from build123d import *

# Parameters (mm, degrees)
CUT_EXTRUDE1_DEPTH           = 10
CUT_REVOLVE1_ANGLE           = 157.5
CUT_REVOLVE1_OTHER_WAY_ANGLE = 157.5


with BuildPart() as part:
    # Sketch3 → Revolve1 (revolve)
    with BuildSketch(Plane.XY, mode=Mode.PRIVATE) as revolve1_sk:
        with BuildLine():
            Line((1.25, 0), (1.25, 9))
            ThreePointArc((1.25, 9), (0, 9.690197618), (-1.25, 9))
            Line((-1.25, 9), (-1.25, 0))
            Line((-1.25, 0), (1.25, 0))
        make_face()
    revolve(revolve1_sk.sketch.rotate(Axis((-1.25, 0, 0), (1, 0, 0)), 180), axis=Axis((-1.25, 0, 0), (1, 0, 0)))

    # Sketch4 → Cut-Extrude1 (cut)
    # profile 1 of 2: a face of its own
    with BuildSketch(Plane(origin=(1.25, 0, 0), x_dir=(0, 0, -1), z_dir=(1, 0, 0))):
        with BuildLine():
            Line((1.322875656, 1.5), (-1.322875656, 1.5))
            ThreePointArc((-1.322875656, 1.5), (0, -2), (1.322875656, 1.5))
        make_face()
        with BuildLine():
            ThreePointArc((-1.118033989, 1), (0, -1.5), (1.118033989, 1))
            Line((1.118033989, 1), (-1.118033989, 1))
        make_face(mode=Mode.SUBTRACT)
    # profile 2 of 2: a face of its own
    with BuildSketch(Plane(origin=(1.25, 0, 0), x_dir=(0, 0, -1), z_dir=(1, 0, 0))):
        with BuildLine():
            Line((1.118033989, 1), (-1.118033989, 1))
            ThreePointArc((-1.118033989, 1), (0, -1.5), (1.118033989, 1))
        make_face()
    extrude(amount=-CUT_EXTRUDE1_DEPTH, mode=Mode.SUBTRACT)

    # Sketch7 → Cut-Revolve1 (revolve, cut)
    with BuildSketch(Plane.XY):
        with BuildLine():
            ThreePointArc((-1.25, 9), (0, 9.690197618), (1.25, 9))
            Line((1.25, 9), (1.25, 3))
            Line((1.25, 3), (-1.25, 3))
            Line((-1.25, 3), (-1.25, 9))
        make_face()
    revolve(axis=Axis((-1.25, 0, 0), (1, 0, 0)), revolution_arc=CUT_REVOLVE1_ANGLE, mode=Mode.SUBTRACT)

    # Sketch7 → Cut-Revolve1 other way (revolve, cut)
    with BuildSketch(Plane.XY):
        with BuildLine():
            ThreePointArc((-1.25, 9), (0, 9.690197618), (1.25, 9))
            Line((1.25, 9), (1.25, 3))
            Line((1.25, 3), (-1.25, 3))
            Line((-1.25, 3), (-1.25, 9))
        make_face()
    revolve(axis=Axis((-1.25, 0, 0), (-1, 0, 0)), revolution_arc=CUT_REVOLVE1_OTHER_WAY_ANGLE, mode=Mode.SUBTRACT)


solid = part.part
Read the model definition and answer for the solid it produces. Units are mm, in the model's axes. A direction names the side the tool comes from. Coordinates: 2 decimals unless noted, no trailing zeros. Write each loop counter-clockwise with the first axis right and the second up, starting at its lowest first coordinate (ties: lowest second). Pieces come first, ordered by that corner, then holes. Notation, with made-up numbers: (-12.75, 42) - (44.25, 42) arc R15 cw to (44.25, 70) - close; hole circle Ø7 at (47.5, 40). An arc over 180 degrees is marked (long way). One line per question, with ' | ' between items.
Q1. Find section B-B, the plane y = 0. Write down the section's boundary in (x, z), plus the area to 3 significant figures.
Result set:
outline: (-1.25, -3) - (1.25, -3) - (1.25, -2) - (-1.25, -2) - close; (-1.25, 2) - (1.25, 2) - (1.25, 3) - (-1.25, 3) - close | area: 5.00 mm^2
Q2. Find section C-C, the plane x = 0.45. Write down the section's boundary in (y, z), plus the area to 3 significant figures.
Result set:
outline: (-8.89, -3.68) - (-2.77, -1.15) arc R3 ccw (long way) to (-2.77, 1.15) - (-8.89, 3.68) arc R9.62 ccw to start; hole (1.5, -1.32) - (1.5, 1.32) arc R2 ccw (long way) to start | area: 49.4 mm^2
Q3. For faces 1 (the flat face through (0, 1.5, 0)), 2 (the flat face through (0.02, -5.91, -2.45)), 3 (the flat face through (0.02, -5.91, 2.45)), determine the directions among +Z, -Z, +X, -X, +Y, -Y from which every point of the face is accessible in a straight line to the end or side of a thin tool.
Result set:
face 1: +X, -X | face 2: -Z, +X, -X | face 3: +Z, +X, -X
Q4. Consider L1, parallel to Z at x = 0.1, y = 0; L2, parallel to Y at x = 0.7, z = -0.5; L3, parallel to Y at x = -0.95, z = 2.5. Determine where each line is inside the solid, lowest interval first. Write a range as [from, to].
Result set:
L1: [-3, -2], [2, 3] | L2: [-9.5, -1.94], [1.5, 2.96] | L3: [-9, -6.04], [-1.66, 1.66]
Q5. Each of these flat-tipped pins is pushed along its axis until it touches: P1, Ø1.2, axis at x = 0, z = 0.5, coming from the -Y side; P2, Ø1, axis at x = 0.5, y = -5.5, coming from the -Z side. Where does it stop, or does it pass through?
Result set:
P1: y = -9.69 | P2: z = -2.49
Q6. Determine the mould class of faces 4 (the cylindrical face through (0, -2, 0)), 5 (the flat face through (-1.25, -4, 0)) for opening direction Y: +Y half, -Y half, draft (parallel to the pull), parting line (faces both ways), or undercut.
Result set:
face 4: undercut | face 5: draft
Q7. Find section A-A, the plane z = 0. Write down the section's boundary in (x, y), plus the area to 3 significant figures.
Result set:
outline: (-1.25, -9) arc R1.48 ccw to (1.25, -9) - (1.25, -2) - (-1.25, -2) - close; (-1.25, 1.5) - (1.25, 1.5) - (1.25, 3) - (-1.25, 3) - close | area: 22.5 mm^2
Q8. Find section D-D, the plane x = -0.1. Write down the section's boundary in (y, z).
Result set:
outline: (-8.95, -3.71) - (-2.77, -1.15) arc R3 ccw (long way) to (-2.77, 1.15) - (-8.95, 3.71) arc R9.69 ccw to start; hole (1.5, -1.32) - (1.5, 1.32) arc R2 ccw (long way) to start
